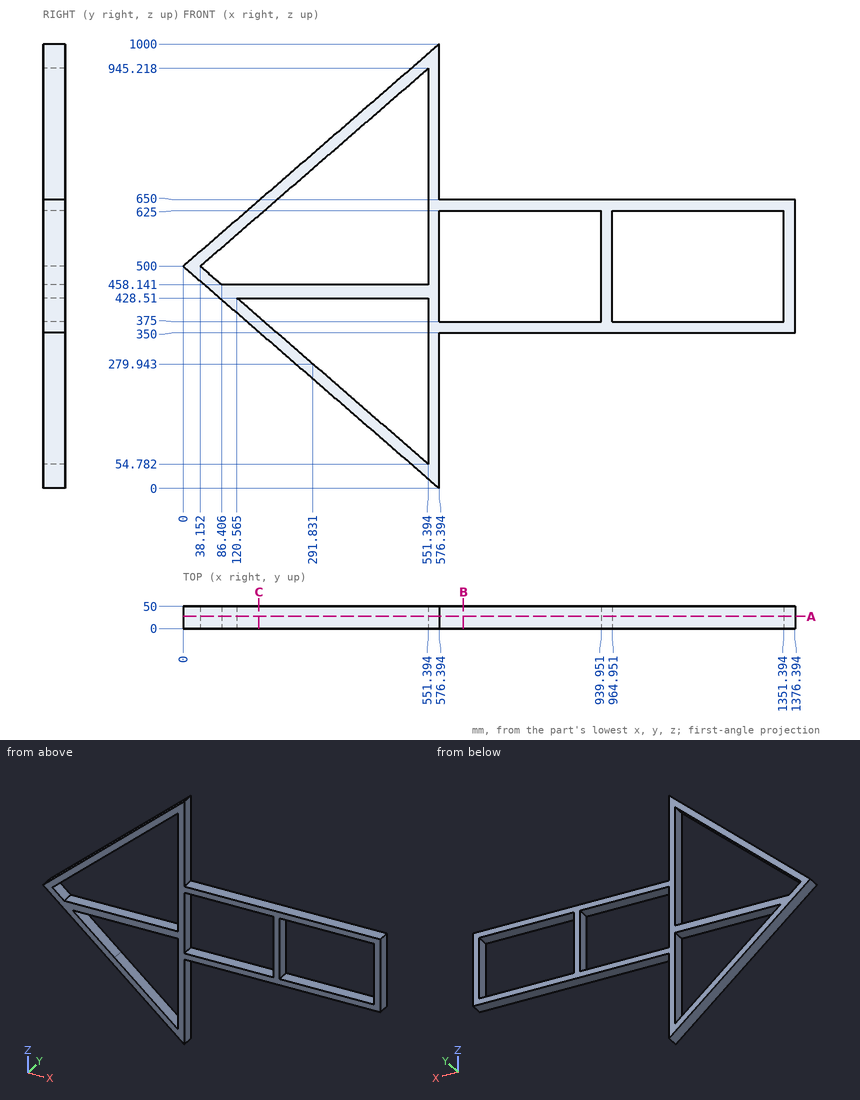
Input: dimensioned drawing with shaded views. Units: mm. Origin: part minimum x, y, z. Coordinates: 2 decimals unless noted, no trailing zeros. Loops run counter-clockwise (first coordinate to the right, second up) from the corner with the lowest first, then second, coordinate; pieces in that order, holes last. Notation, with made-up numbers: (24, 21.25) - (65, 21.25) arc R16 ccw to (65, 52.25) - close; hole circle Ø6 at (-35.75, 0). An arc over 180 degrees is marked (long way). One line per question, with ' | ' between items. Start each with the question number.
(1) Cut plane A-A on y = 28. Count the separate pieces of the cut face and the enclosed holes in it, and give its area (3 significant figures).
(2) Cut plane C-C on x = 170. Output: boundary loops of the cut face in (y, z), and give its area (3 significant figures).
(3) First-contact query: pin 1 (15 mm diameter, centred on x = 915, y = 31.5, fed in from -Z); pin 2 (12 mm diameter, centred on y = 22, z = 323.5, fed in from +X); pin 3 (1 mm diameter, centred on x = 465, y = 25, fed in from -Z) (1 decimal). Flat tips, straight axial feed; report the tip coordinate or a pass-through.
(4) Ray query, L1, parallel to Z at x = 1098, y = 38.5; L2, parallel to Z at x = 249, y = 25 (1 decimal); L3, parallel to Z at x = 354, y = 13 (1 decimal). Return the intervals inside material, ascending. Write a range as from..to.
(5) Cut plane B-B on x = 630.5. Output: boundary loops of the cut face in (y, z).
Here are the results:
1) separate pieces: 1 | enclosed holes: 4 | area: 125,000 mm²
2) outline: (0, 352.53) - (50, 352.53) - (50, 385.63) - (0, 385.63) - close; (0, 428.51) - (50, 428.51) - (50, 458.14) - (0, 458.14) - close; (0, 614.37) - (50, 614.37) - (50, 647.47) - (0, 647.47) - close | area: 4,790 mm²
3) pin 1: z = 350 | pin 2: x = 576.39 | pin 3: z = 96.2
4) L1: 350..375, 625..650 | L2: 284..317.1, 428.5..458.1, 682.9..716 | L3: 192.9..226, 428.5..458.1, 774..807.1
5) outline: (0, 350) - (50, 350) - (50, 375) - (0, 375) - close; (0, 625) - (50, 625) - (50, 650) - (0, 650) - close
